Source: CAD feature listing. Evaluate the final solid. Frame: model axes, mm. A direction names the side the tool comes from. Give positions to 0.01 mm unless a question says otherwise; leave off trailing zeros. Loops run counter-clockwise (first coordinate to the right, second up) from the corner with the lowest first, then second, coordinate; pieces in that order, holes last. Notation, with made-up numbers: (19.5, 30.25) -> (26.5, 30.25) arc R15 cw to (26.5, 42.25) -> close; hole circle Ø6 at (-10.75, -16.5). An arc over 180 degrees is marked (long way). Put each result on its own line as item: value.
```python
from build123d import *

# Parameters (mm, degrees)
FILLET_2_R            = 0.2
HOLE_WIZARD_M31_D     = 2.5
HOLE_WIZARD_M31_DEPTH = 4
HOLE_WIZARD_M31_TIP   = 0.751075774
CHAMFER_2_SIZE        = 0.15
CHAMFER_3_SIZE        = 0.2
CHAMFER_6_SIZE        = 0.2


with BuildPart() as part:
    # Эскиз1 → Повернуть1 (revolve)
    with BuildSketch(Plane.XY, mode=Mode.PRIVATE) as revolve_1_sk:
        Polygon((0, 0), (2.45, 0), (2.45, 5.2), (3, 5.2), (3, 6), (0, 6), align=None)
    revolve(revolve_1_sk.sketch.rotate(Axis((0, 0, 0), (0, 1, 0)), 90), axis=Axis((0, 0, 0), (0, 1, 0)))

    # Скругление2
    fillet_2_edges = [part.edges().sort_by_distance(p)[0] for p in [
        (0, 6, 3),
    ]]
    fillet(fillet_2_edges, radius=FILLET_2_R)

    # Отверстие обработанное метчиком M31
    with Locations(Plane(origin=(0, 0, 0), x_dir=(-1, 0, 0), z_dir=(0, -1, 0))):
        with Locations((0, 0)):
            Hole(HOLE_WIZARD_M31_D / 2, depth=HOLE_WIZARD_M31_DEPTH)
            with Locations((0, 0, -(HOLE_WIZARD_M31_DEPTH + HOLE_WIZARD_M31_TIP / 2))):  # 118° drill point
                Cone(0, HOLE_WIZARD_M31_D / 2, HOLE_WIZARD_M31_TIP, mode=Mode.SUBTRACT)

    # Фаска2
    chamfer_2_edges = [part.edges().sort_by_distance(p)[0] for p in [
        (-1.25, 0, 0),
    ]]
    chamfer(chamfer_2_edges, length=CHAMFER_2_SIZE)

    # Эскиз8 → Вырез-Повернуть1 (revolve, cut)
    with BuildSketch(Plane.XY, mode=Mode.PRIVATE) as cut_revolve_1_sk:
        Polygon((2.25, 6), (2.25, 3.419676892), (1.35, 3), (0, 3), (0, 6), align=None)
    revolve(cut_revolve_1_sk.sketch.rotate(Axis((0, 6, 0), (0, -1, 0)), 90), axis=Axis((0, 6, 0), (0, -1, 0)), mode=Mode.SUBTRACT)

    # Эскиз9 → Повернуть3 (revolve)
    with BuildSketch(Plane.XY, mode=Mode.PRIVATE) as revolve_3_sk:
        with BuildLine():
            Line((-2.45, 4.2), (-2.45, 3.08))
            ThreePointArc((-2.45, 3.08), (-3.01, 3.64), (-2.45, 4.2))
        make_face()
    revolve(revolve_3_sk.sketch.rotate(Axis((0, 0, 0), (0, 1, 0)), 270), axis=Axis((0, 0, 0), (0, 1, 0)))

    # Фаска3
    chamfer_3_edges = [part.edges().sort_by_distance(p)[0] for p in [
        (0, 0, 2.45),
    ]]
    chamfer(chamfer_3_edges, length=CHAMFER_3_SIZE)

    # Фаска6
    chamfer_6_edges = [part.edges().sort_by_distance(p)[0] for p in [
        (0, 6, -2.25),
    ]]
    chamfer(chamfer_6_edges, length=CHAMFER_6_SIZE)


solid = part.part
```
(1) Reachability of faces 1 (the cylindrical face through (-0.27, 1.59, 1.22)), 2 (the cylindrical face through (-0.9, 5.5, -2.86)), 3 (the cylindrical face through (-1.656, 1.66, 1.806)) from +Z, -Z, +X, -X, +Y, -Y: full face, straight path, thin tool, end or side. Return the list, or none.
Calculated:
face 1: +Y, -Y
face 2: +Y
face 3: -Y
(2) Section D-D on y = 2.85. Return loops of the section in (x, z), then the cut area to 3 significant figures.
Calculated:
outline: circle Ø4.9 at (0, 0); hole circle Ø2.5 at (0, 0)
area: 13.9 mm²
(3) Line query: probe 1 along X at (y, z) = (4.25, 0); probe 2 along X at (y, z) = (0.8, 0); probe 3 along Y at (x, z) = (2.5, -1.25). Output: solid intervals per line, ascending. Write a range as from..to.
Calculated:
probe 1: x = -2.45..-2.25, 2.25..2.45
probe 2: x = -2.45..-1.25, 1.25..2.45
probe 3: y = 3.2..4.08, 5.2..6
(4) First-contact query: P1, Ø1, axis at y = 2, z = -2, coming from the -X side; P2, Ø3, axis at x = -0.5, y = 5.5, coming from the +Z side; P3, Ø1.8, axis at x = 0.5, z = 1, coming from the -Y side; P4, Ø2, axis at x = -0.5, z = -0.5, coming from the +Y side. Flat tips, straight axial feed; report the tip coordinate or a pass-through.
Calculated:
P1: stops at x = -1.94
P2: stops at z = 3
P3: stops at y = 0
P4: stops at y = 3.17
(5) Section C-C on y = 4.3. Return loops of the section in (x, z).
Calculated:
outline: circle Ø4.9 at (0, 0); hole circle Ø4.5 at (0, 0)
(6) Draft query along X for faces 4 (the flat face through (1.5, 0, 0.5)), 5 (the cylindrical face through (-1.52, 4.59, -1.66)), 6 (the cylindrical face through (-1.656, 4.707, 1.806)). Return one class per face: released by +X, released by -X, zero draft, split by the parting line, or undercut.
Calculated:
face 4: zero draft
face 5: undercut
face 6: split by the parting line
